Part model, mm, in its own coordinate system. Face numbers are marked on the shaded views. A direction names the side the tool comes from. Give positions to 0.01 mm unless a question says otherwise; leave off trailing zeros. Loops run counter-clockwise (first coordinate to the right, second up) from the corner with the lowest first, then second, coordinate; pieces in that order, holes last. Notation, with made-up numbers: M -19.5,85 L 0.5,85 A33 cw 0.5,115 Z; hole C 45.25,-39 d5. An arc over 180 degrees is marked long. Answer in a Markdown table with one row per item.
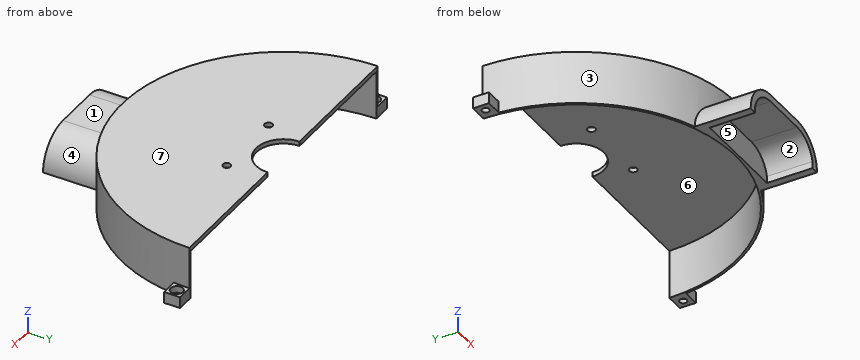
from build123d import *

# Parameters (mm, degrees)
BOSS_EXTRUDE1_DEPTH = 21.5
BOSS_EXTRUDE2_DEPTH = 2
SKETCH3_W           = 50
SKETCH3_H           = 20
BOSS_EXTRUDE3_DEPTH = 15
SKETCH8_R           = 1.6
BOSS_EXTRUDE5_DEPTH = 5
SKETCH10_R          = 2.7
SKETCH10_R_2        = 2.6
CUT_EXTRUDE5_DEPTH  = 3
FILLET2_R           = 15
SKETCH11_W          = 43.237900078
SKETCH11_H          = 3
CUT_EXTRUDE7_DEPTH  = 20
SKETCH13_R          = 1.7
CUT_EXTRUDE8_DEPTH  = 10
SKETCH14_R          = 12
CUT_EXTRUDE9_DEPTH  = 10


with BuildPart() as part:
    # Sketch1 → Boss-Extrude1 (new body)
    with BuildSketch(Plane.XY):
        with BuildLine():
            Line((71, 0), (70, 0))
            ThreePointArc((70, 0), (0, -70), (-70, 0))
            Line((-70, 0), (-71, 0))
            ThreePointArc((-71, 0), (0, -71), (71, 0))
        make_face()
    extrude(amount=BOSS_EXTRUDE1_DEPTH)

    # Sketch2 → Boss-Extrude2 (add)
    with BuildSketch(Plane.XY.offset(21.5)):
        with BuildLine():
            Line((71, 0), (70, 0))
            ThreePointArc((70, 0), (0, -70), (-70, 0))
            Line((-70, 0), (-71, 0))
            ThreePointArc((-71, 0), (0, -71), (71, 0))
        make_face()
        with BuildLine():
            Line((-21.5, 0), (-70, 0))
            ThreePointArc((-70, 0), (0, -70), (70, 0))
            Line((70, 0), (21.5, 0))
            Line((21.5, 0), (-21.5, 0))
        make_face()
    extrude(amount=BOSS_EXTRUDE2_DEPTH)

    # Sketch3 → Boss-Extrude3 (add)
    with BuildSketch(Plane(origin=(0, 0, 0), x_dir=(-1, 0, 0), z_dir=(0, 0, -1))):
        with BuildLine():
            Line((-25, -66.452990903), (-25, -71))
            Line((-25, -71), (0, -71))
            ThreePointArc((0, -71), (-12.705070757, -69.853999006), (-25, -66.452990903))
        make_face()
        with BuildLine():
            ThreePointArc((25, -66.452990903), (12.705070757, -69.853999006), (0, -71))
            Line((0, -71), (25, -71))
            Line((25, -71), (25, -66.452990903))
        make_face()
        with Locations((0, -81)):
            Rectangle(SKETCH3_W, SKETCH3_H)
    extrude(amount=-BOSS_EXTRUDE3_DEPTH)

    # Sketch8 → Boss-Extrude5 (add)
    # profile 1 of 2: a face of its own
    with BuildSketch(Plane(origin=(0, 0, 0), x_dir=(-1, 0, 0), z_dir=(0, 0, -1))):
        with BuildLine():
            ThreePointArc((-70.654086931, -7), (-70.913469003, -3.504270818), (-71, 0))
            Line((-71, 0), (-78, 0))
            Line((-78, 0), (-78, -7))
            Line((-78, -7), (-70.654086931, -7))
        make_face()
        with Locations((-74.5, -3.5)):
            Circle(SKETCH8_R, mode=Mode.SUBTRACT)
    # profile 2 of 2: a face of its own
    with BuildSketch(Plane(origin=(0, 0, 0), x_dir=(-1, 0, 0), z_dir=(0, 0, -1))):
        with BuildLine():
            Line((78, 0), (71, 0))
            ThreePointArc((71, 0), (70.913469003, -3.504270818), (70.654086931, -7))
            Line((70.654086931, -7), (78, -7))
            Line((78, -7), (78, 0))
        make_face()
        with Locations(Location((74.5, -3.5, 0), (0, 0, 180))):
            Circle(SKETCH8_R, mode=Mode.SUBTRACT)
    extrude(amount=-BOSS_EXTRUDE5_DEPTH)

    # Sketch10 → Cut-Extrude5 (cut)
    with BuildSketch(Plane.XY.offset(5)):
        with Locations((74.5, -3.5)):
            Circle(SKETCH10_R)
        with Locations((-74.5, -3.5)):
            Circle(SKETCH10_R_2)
    extrude(amount=-CUT_EXTRUDE5_DEPTH, mode=Mode.SUBTRACT)

    # Fillet2
    fillet2_edges = [part.edges().sort_by_distance(p)[0] for p in [
        (-25, -78.726495452, 15),
        (25, -78.726495452, 15),
    ]]
    fillet(fillet2_edges, radius=FILLET2_R - 0.0001)  # a hair under: the kernel refuses the full size

    # Sketch11 → Cut-Extrude7 (cut)
    with BuildSketch(Plane.XZ.offset(91)):
        with Locations((0, 1.5)):
            Rectangle(SKETCH11_W, SKETCH11_H)
        with BuildLine():
            Line((-21.618950039, 3), (21.618950039, 3))
            ThreePointArc((21.618950039, 3), (17.348469228, 9.486832981), (10, 12))
            Line((10, 12), (-10, 12))
            ThreePointArc((-10, 12), (-17.348469228, 9.486832981), (-21.618950039, 3))
        make_face()
    extrude(amount=-CUT_EXTRUDE7_DEPTH, mode=Mode.SUBTRACT)

    # Sketch13 → Cut-Extrude8 (cut)
    with BuildSketch(Plane.XY.offset(23.5)):
        with Locations((-15.75, -15.75)):
            Circle(SKETCH13_R)
        with Locations((15.75, -15.75)):
            Circle(SKETCH13_R)
    extrude(amount=-CUT_EXTRUDE8_DEPTH, mode=Mode.SUBTRACT)

    # Sketch14 → Cut-Extrude9 (cut)
    with BuildSketch(Plane.XY.offset(23.5)):
        Circle(SKETCH14_R)
    extrude(amount=-CUT_EXTRUDE9_DEPTH, mode=Mode.SUBTRACT)


solid = part.part
(1) Which spindle directions (+Z, -Z, +X, -X, +Y, -Y) get a long thin tool onto all of the face, cutting with end or side? Do the marked faces 4, 5, 6 and 7. Say none if no direction does.
Recorded:
| item | result |
|---|---|
| face 4 | +Z, +X, -Y |
| face 5 | -Z, -Y |
| face 6 | -Z, +Y |
| face 7 | +Z, +X, -X, +Y, -Y |
(2) Pull direction X, two halves, no side cores. Call the marked faces 1, 2 and 3: +X half, -X half, draft (parallel to the pull), parting line (faces both ways), or undercut.
Recorded:
| item | result |
|---|---|
| face 1 | draft |
| face 2 | undercut |
| face 3 | parting line |
(3) Saw through at A-A (x = 15.75). Write the cut outline in (y, z).
Recorded:
| item | result |
|---|---|
| outline | M -91,10.53 L -71,10.53 L -71,0 L -68.21,0 L -68.21,21.5 L -17.45,21.5 L -17.45,23.5 L -69.23,23.5 L -69.23,13.85 L -91,13.85 Z; M -14.05,21.5 L 0,21.5 L 0,23.5 L -14.05,23.5 Z |
(4) Saw through at B-B (y = -15.75). Write the cut outline in (x, z), plus the area to 3 significant figures.
Recorded:
| item | result |
|---|---|
| outline | M -69.23,0 L -68.21,0 L -68.21,21.5 L -17.45,21.5 L -17.45,23.5 L -69.23,23.5 Z; M -14.05,21.5 L 14.05,21.5 L 14.05,23.5 L -14.05,23.5 Z; M 17.45,21.5 L 68.21,21.5 L 68.21,0 L 69.23,0 L 69.23,23.5 L 17.45,23.5 Z |
| area | 307 mm^2 |
(5) Pin check, flat tips, straight feed: pin 1 Ø6 at (x, z) = (-25.5, 7.5) entering from +Y; pin 2 Ø8 at (y, z) = (-67.5, 7.5) entering from -X; pin 3 Ø6 at (x, y) = (-0.5, -78) entering from +Z. Stop position of each tip, or through.
Recorded:
| item | result |
|---|---|
| pin 1 | stops at y = -63.94 |
| pin 2 | stops at x = -31.76 |
| pin 3 | stops at z = 15 |
(6) Drill centre lines: line 1 along Y through (x, z) = (74.5, 4.15); line 2 along Y through (x, z) = (-74.5, 2.95); line 3 along Z through (x, y) = (30, -26.5). Where is each one in solid material? Low to high.
Recorded:
| item | result |
|---|---|
| line 1 | y = -7 to -6.2, -0.8 to 0 |
| line 2 | y = -7 to -6.1, -0.9 to 0 |
| line 3 | z = 21.5 to 23.5 |
(7) Saw through at C-C (z = 7.25). Write the cut outline in (x, y).
Recorded:
| item | result |
|---|---|
| outline | M -71,0 A71 ccw -23.13,-67.13 L -23.13,-91 L -19.56,-91 L -19.56,-71 L 19.56,-71 L 19.56,-91 L 23.13,-91 L 23.13,-67.13 A71 ccw 71,0 L 70,0 A70 cw -70,0 Z |
